Verification items for the finished model (mm, model axes). Face numbers are marked on the shaded views. A direction names the side the tool comes from. Round coordinates to 2 decimals unless told otherwise and drop trailing zeros. Write each loop counter-clockwise with the first axis right and the second up, starting at its lowest first coordinate (ties: lowest second). Pieces come first, ordered by that corner, then holes. Notation, with made-up numbers: M -24,33 L 31,33 A22 cw 31,41 Z; hole C -3.5,-24.75 d3. An arc over 180 degrees is marked long. Answer in a Markdown table with one row per item. Add a question column.
1. Set-up check for the marked faces 1, 2, 3 and 4: record each of +Z, -Z, +X, -X, +Y, -Y from which the full face is reachable in a straight line by a thin tool's end or side.
2. Go/stop test with flat-tipped pins: pin 1 Ø7 at (x, z) = (-2, -3) entering from +Y; pin 2 Ø1.5 at (x, y) = (-5.5, 16.5) entering from +Z; pin 3 Ø10 at (x, y) = (4.5, 12) entering from +Z; pin 4 Ø8.5 at (x, y) = (2.5, 33) entering from +Z. Record where each tip stops, or that it passes through.
3. Material ranges on probe 1 along X at (y, z) = (30, 22.4); probe 2 along X at (y, z) = (30, 24.2); probe 3 along Y at (x, z) = (0.5, 21.5), recorded low to high.
4. Sectioned sample at A-A on z = 22.5. Record the cut outline in (x, y).
5. Sectioned sample at C-C on z = 15. Record the cut outline in (x, y), plus the area to 3 significant figures.
6. Sectioned sample at B-B on y = 10.5. Record the cut outline in (x, z), plus the area to 3 significant figures.
7. Draft check along Z on the marked faces 5, 6 and 7. Enter one of: pulls with the +Z half, pulls with the -Z half, needs draft (parallel to the pull), parting line crosses it, or undercut.
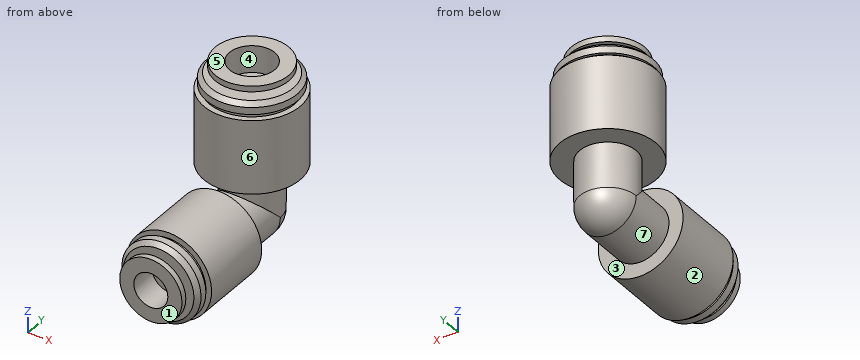
```python
from build123d import *
from build123d.topology import SkipClean

# Parameters (mm, degrees)
SKETCH_3_R      = 5
EXTRUDE_2_DEPTH = 8
SKETCH_4_R      = 8.5
EXTRUDE_3_DEPTH = 13
EXTRUDE_START   = 3.5
SKETCH_7_R      = 5
EXTRUDE_4_DEPTH = 3.5
SKETCH_8_R      = 7.5
EXTRUDE_6_DEPTH = 13


with BuildPart() as part:
    # Эскиз2 → Повернуть1 (revolve)
    with BuildSketch(Plane.XY, mode=Mode.PRIVATE) as revolve_1_sk:
        with BuildLine():
            Line((0, 25), (0, 35))
            ThreePointArc((0, 35), (3.535533906, 33.535533906), (5, 30))
            Line((5, 30), (5, 25))
            Line((5, 25), (0, 25))
        make_face()
    revolve(revolve_1_sk.sketch.rotate(Axis((0, 25, 0), (0, 1, 0)), 90), axis=Axis((0, 25, 0), (0, 1, 0)))

    # Эскиз3 → Бобышка-Вытянуть2 (add)
    with SkipClean():  # the faces are left unmerged after this step: merging them gives an invalid solid
        with BuildSketch(Plane.XY):
            with Locations((0, 30)):
                Circle(SKETCH_3_R)
        extrude(amount=EXTRUDE_2_DEPTH)

    # Эскиз4 → Бобышка-Вытянуть3 (add)
    with SkipClean():  # the faces are left unmerged after this step: merging them gives an invalid solid
        with BuildSketch(Plane.XY.offset(8)):
            with Locations(Location((0, 30, 0), (0, 0, 180))):
                Circle(SKETCH_4_R)
        extrude(amount=EXTRUDE_3_DEPTH)

    # Эскиз7 → Бобышка-Вытянуть4 (add)
    with BuildSketch(Plane.XZ.offset(-25).offset(EXTRUDE_START)):
        with Locations(Location((0, 0, 0), (0, 0, 270))):
            Circle(SKETCH_7_R)
    extrude(amount=-EXTRUDE_4_DEPTH)

    # Эскиз8 → Бобышка-Вытянуть6 (add)
    with BuildSketch(Plane.XZ.offset(-21.5)):
        with Locations(Location((0, 0, 0), (0, 0, 90))):
            Circle(SKETCH_8_R)
    extrude(amount=EXTRUDE_6_DEPTH)

    # Эскиз9 → Повернуть5 (revolve)
    with BuildSketch(Plane(origin=(0, 0, 0), x_dir=(0, 0, -1), z_dir=(1, 0, 0)), mode=Mode.PRIVATE) as revolve_5_sk:
        Polygon((5.5, 4.75), (3.5, 4.75), (3.5, 5.75), (6.25, 5.75), (7, 6.5), (7, 7.75), (6.5, 7.75), (6.5, 8.5), (3, 8.5), (3, 3.75), (5.5, 3.75), align=None)
    revolve(revolve_5_sk.sketch.rotate(Axis((0, 8.5, 0), (0, -1, 0)), 180), axis=Axis((0, 8.5, 0), (0, -1, 0)))

    # Эскиз5 → Повернуть6 (revolve)
    with BuildSketch(Plane(origin=(0, 0, 0), x_dir=(0, 0, -1), z_dir=(1, 0, 0)), mode=Mode.PRIVATE) as revolve_6_sk:
        Polygon((-24.75, 23.5), (-24.75, 25.5), (-23.75, 25.5), (-23.75, 22.75), (-23, 22), (-21.75, 22), (-21.75, 22.5), (-21, 22.5), (-21, 26), (-25.75, 26), (-25.75, 23.5), align=None)
    revolve(revolve_6_sk.sketch.rotate(Axis((0, 30, 21), (0, 0, 1)), 180), axis=Axis((0, 30, 21), (0, 0, 1)))


solid = part.part
```
Geometry check:
| question | item | result |
|---|---|---|
| 1 | face 1 | +Z, -Z, +X, -X, -Y |
| 1 | face 2 | -Y |
| 1 | face 3 | none |
| 1 | face 4 | +Z |
| 2 | pin 1 | stops at y = 35 |
| 2 | pin 2 | stops at z = 5.8 |
| 2 | pin 3 | stops at z = 7.5 |
| 2 | pin 4 | stops at z = 25.75 |
| 3 | probe 1 | x = -8 to -4, 4 to 8 |
| 3 | probe 2 | x = -4.5 to -4, 4 to 4.5 |
| 3 | probe 3 | y = 22.52 to 26.03, 33.97 to 37.48 |
| 4 | outline | C 0,30 d16; hole C 0,30 d8 |
| 5 | outline | C 0,30 d17 |
| 5 | area | 227 mm2 |
| 6 | outline | C 0,0 d15 |
| 6 | area | 177 mm2 |
| 7 | face 5 | pulls with the +Z half |
| 7 | face 6 | needs draft |
| 7 | face 7 | undercut |
